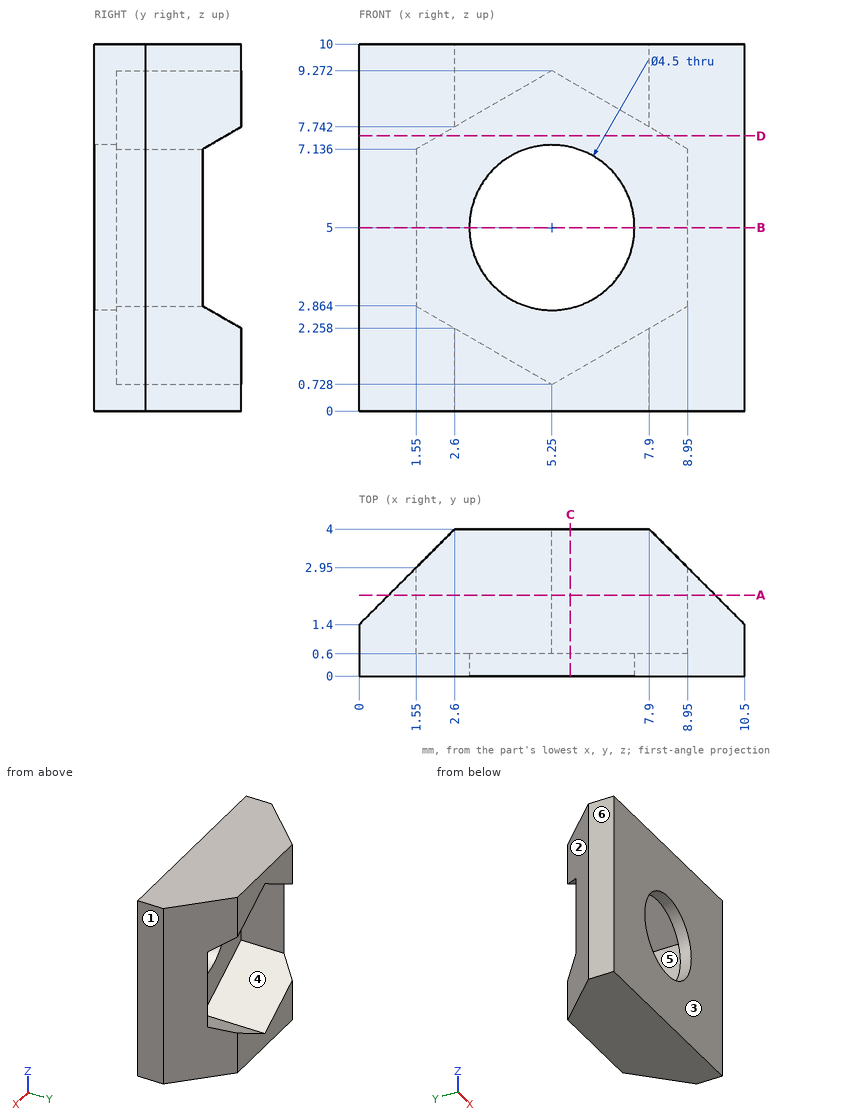
Verification items for this drawing (mm, ordinates from the low corner). A direction names the side the tool comes from. Give positions to 0.01 mm unless a question says otherwise; leave off trailing zeros. Write each loop counter-clockwise with the first axis right and the second up, starting at its lowest first coordinate (ties: lowest second). Pieces come first, ordered by that corner, then holes. Notation, with made-up numbers: (15, 44.5) - (21, 44.5) arc R33 cw to (21, 74.5) - close; hole circle Ø3 at (-4.5, -5). An arc over 180 degrees is marked (long way). Answer as a JSON object with one key per item and string values. Group by question number.
1) Release check for a two-part mould opening along X. For the marked faces 1, 2, 3 and 4 record: pulls with the +X half, pulls with the -X half, needs draft (parallel to the pull), parting line crosses it, or undercut.
2) Access from +Z, -Z, +X, -X, +Y, -Y to the whole of each face (thin tool, end or side, straight path). Record for the marked faces 5 and 6.
3) Sectioned sample at B-B (z = 5). Record the cut outline in (x, y).
4) Depth check by flat-ended pin: P1, Ø1, axis at x = 9, z = 4.5, coming from the +Y side; P2, Ø1.5, axis at x = 1.5, z = 1, coming from the +Y side. Enter the tip coordinate at first touch or a pass-through.
5) Sectioned sample at D-D (z = 7.5). Record the cut outline in (x, y).
6) Sectioned sample at C-C (x = 5.75). Record the cut outline in (y, z), then the cut area to 3 significant figures.
7) Thickness scan on probe 1 along Z at (x, y) = (5.25, 0.25); probe 2 along Y at (x, z) = (7.5, 5.75); probe 3 along Z at (x, y) = (2.25, 3.05). Record the ranges inside material, lowest first. Write a range as from..to.
8) Sectioned sample at A-A (y = 2.2). Record the cut outline in (x, z).
Geometry results:
{
 "1": {"face 1": "pulls with the +X half", "face 2": "pulls with the -X half", "face 3": "needs draft", "face 4": "undercut"},
 "2": {"face 5": "+Y", "face 6": "+Z, -Z, -X, +Y, -Y"},
 "3": {"outline": "(0, 0) - (3, 0) - (3, 0.6) - (1.55, 0.6) - (1.55, 2.95) - (0, 1.4) - close; (7.5, 0) - (10.5, 0) - (10.5, 1.4) - (8.95, 2.95) - (8.95, 0.6) - (7.5, 0.6) - close"},
 "4": {"P1": "stops at y = 2.95", "P2": "stops at y = 3.65"},
 "5": {"outline": "(0, 0) - (10.5, 0) - (10.5, 1.4) - (8.32, 3.58) - (8.32, 0.6) - (2.18, 0.6) - (2.18, 3.58) - (0, 1.4) - close"},
 "6": {"outline": "(0, 0) - (4, 0) - (4, 1.02) - (0.6, 1.02) - (0.6, 2.81) - (0, 2.81) - close; (0, 7.19) - (0.6, 7.19) - (0.6, 8.98) - (4, 8.98) - (4, 10) - (0, 10) - close", "area": "10.3 mm^2"},
 "7": {"probe 1": "z = 0..2.75, 7.25..10", "probe 2": "y = 0..0.6", "probe 3": "z = 0..2.46, 7.54..10"},
 "8": {"outline": "(0.8, 0) - (9.7, 0) - (9.7, 10) - (0.8, 10) - close; hole (1.55, 2.86) - (5.25, 0.73) - (8.95, 2.86) - (8.95, 7.14) - (5.25, 9.27) - (1.55, 7.14) - close"}
}
